```python
from build123d import *

# Parameters (mm, degrees)
SKETCH_1_W          = 50
SKETCH_1_H          = 50
EXTRUDE_1_DEPTH     = 6
CUT_EXTRUDE_1_REACH = 37.861
SKETCH_2_R          = 2.1
CUT_EXTRUDE_2_REACH = 37.861
SKETCH_3_R          = 2.1


with BuildPart() as part:
    # 草图1 → 凸台-拉伸1 (new body)
    with BuildSketch(Plane(origin=(0, 0, 0), x_dir=(1, 0, 0), z_dir=(0, 1, 0))):
        Rectangle(SKETCH_1_W, SKETCH_1_H)
    extrude(amount=EXTRUDE_1_DEPTH)

    # 草图2 → 切除-拉伸1 (cut, up to next)
    with BuildSketch(Plane(origin=(0, 6, 0), x_dir=(1, 0, 0), z_dir=(0, 1, 0)), mode=Mode.PRIVATE) as cut_extrude_1_sk1:
        with Locations(Location((-15, 12.9, 0), (0, 0, 270))):
            Circle(SKETCH_2_R)
    cut_extrude_1_tool1 = extrude(cut_extrude_1_sk1.sketch, amount=-CUT_EXTRUDE_1_REACH, mode=Mode.PRIVATE) & part.part
    # 草图2 → 切除-拉伸1 (cut, up to next)
    with BuildSketch(Plane(origin=(0, 6, 0), x_dir=(1, 0, 0), z_dir=(0, 1, 0)), mode=Mode.PRIVATE) as cut_extrude_1_sk2:
        with Locations(Location((15, 12.9, 0), (0, 0, 270))):
            Circle(SKETCH_2_R)
    cut_extrude_1_tool2 = extrude(cut_extrude_1_sk2.sketch, amount=-CUT_EXTRUDE_1_REACH, mode=Mode.PRIVATE) & part.part
    add(cut_extrude_1_tool1.solids().sort_by_distance((-15, 6, -12.9))[0], mode=Mode.SUBTRACT)
    add(cut_extrude_1_tool2.solids().sort_by_distance((15, 6, -12.9))[0], mode=Mode.SUBTRACT)

    # 草图3 → 切除-拉伸2 (cut, up to next)
    with BuildSketch(Plane(origin=(0, 6, 0), x_dir=(1, 0, 0), z_dir=(0, 1, 0)), mode=Mode.PRIVATE) as cut_extrude_2_sk1:
        with Locations(Location((15, -16.9, 0), (0, 0, 270))):
            Circle(SKETCH_3_R)
    cut_extrude_2_tool1 = extrude(cut_extrude_2_sk1.sketch, amount=-CUT_EXTRUDE_2_REACH, mode=Mode.PRIVATE) & part.part
    add(cut_extrude_2_tool1.solids().sort_by_distance((15, 6, 16.9))[0], mode=Mode.SUBTRACT)


solid = part.part
```
Geometry: final body of the model. Coordinates: model frame, mm. Round coordinates to 2 decimals unless told otherwise and drop trailing zeros. Order: outer loops, then holes, each group sorted by start corner. A loop starts at its lowest first (then second) coordinate and runs counter-clockwise, first axis right, second up. Notation, with made-up numbers: (1.25, 19.25) - (44.25, 19.25) arc R25 ccw to (44.25, 55.25) - close; hole circle Ø7 at (82, -30.75). An arc over 180 degrees is marked (long way). Use CSV: the item, a comma, the result in double quotes. Start each with the question number.
Q1. Section query D-D (x = -15). Return loops of the section in (y, z).
Q2. Mould query, pull axis Z, two halves, no side actions, for faces 1 (the face through (-25, 3, 0)), 2 (the face through (15.631, 3.042, 18.903)), 3 (the face through (0, 3, 25)). Classes: +Z half, -Z half, draft (parallel to the pull), parting line (faces both ways), or undercut.
Q3. Section query B-B (z = -12.9). Return loops of the section in (x, y).
Q4. Section query C-C (z = 16.9). Return loops of the section in (x, y).
Q5. Material intervals for line 1 along X through (y, z) = (3.5, -12.9); line 2 along X through (y, z) = (2.55, -14); line 3 along X through (y, z) = (1.5, 16.9), sorted ascending. Write a range as from..to.
Q6. Section query A-A (x = 15). Return loops of the section in (y, z), and give its area (3 significant figures).
Result set:
1,outline,"(0, -25) - (6, -25) - (6, -15) - (0, -15) - close; (0, -10.8) - (6, -10.8) - (6, 25) - (0, 25) - close"
2,face 1,"draft"
2,face 2,"undercut"
2,face 3,"+Z half"
3,outline,"(-25, 0) - (-17.1, 0) - (-17.1, 6) - (-25, 6) - close; (-12.9, 0) - (12.9, 0) - (12.9, 6) - (-12.9, 6) - close; (17.1, 0) - (25, 0) - (25, 6) - (17.1, 6) - close"
4,outline,"(-25, 0) - (12.9, 0) - (12.9, 6) - (-25, 6) - close; (17.1, 0) - (25, 0) - (25, 6) - (17.1, 6) - close"
5,line 1,"x = -25..-17.1, -12.9..12.9, 17.1..25"
5,line 2,"x = -25..-16.79, -13.21..13.21, 16.79..25"
5,line 3,"x = -25..12.9, 17.1..25"
6,outline,"(0, -25) - (6, -25) - (6, -15) - (0, -15) - close; (0, -10.8) - (6, -10.8) - (6, 14.8) - (0, 14.8) - close; (0, 19) - (6, 19) - (6, 25) - (0, 25) - close"
6,area,"250 mm2"
